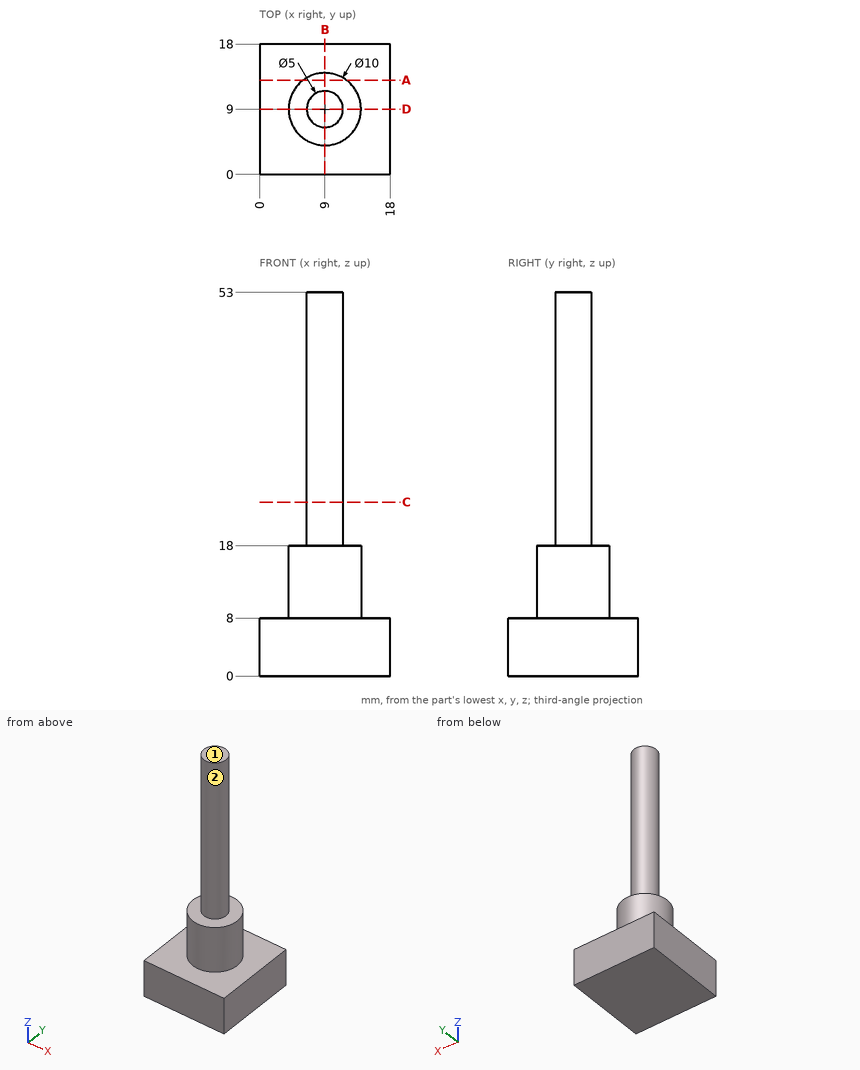
Study the drawing (mm; zero at the part's minimum x, y, z) and answer. A direction names the side the tool comes from. Coordinates: 2 decimals unless noted, no trailing zeros. Loops run counter-clockwise (first coordinate to the right, second up) from the corner with the lowest first, then second, coordinate; pieces in that order, holes last. Notation, with made-up numbers: M -37,-10 L 19,-10 A21 ccw 19,25 Z; hole C -17,16.25 d7. An arc over 180 degrees is marked long. Answer as a JSON object with one key per item and string values. Group by question number.
Item 1: Which of the six approach directions +Z, -Z, +X, -X, +Y, -Y give full straight-line access (tool end or side, diameter ignored) to the marked faces 1 and 2?
Item 2: Section C-C (z = 24) is taken. Write down the section's boundary in (x, y), and give its area (3 significant figures).
Item 3: Section A-A (y = 13) is taken. Write down the section's boundary in (x, z).
Item 4: Each of these flat-tipped pins is pushed along its axis until it touches: P1, Ø4, axis at x = 14, z = 30.5, coming from the +Y side; P2, Ø2, axis at x = 12, z = 15, coming from the -Y side; P3, Ø3, axis at y = 8.5, z = 10, coming from the +X side. Where does it stop, or does it pass through?
Item 5: Section B-B (x = 9) is taken. Write down the section's boundary in (y, z), and give its area (3 significant figures).
Item 6: Consider L1, parallel to Z at x = 10.75, y = 2.5; L2, parallel to Y at x = 9, z = 16; L3, parallel to Z at x = 13.5, y = 8. Determine where each line is inside the solid, lowest interval first.
Solved:
{
 "1": {"face 1": "+Z, +X, -X, +Y, -Y", "face 2": "+Z"},
 "2": {"outline": "C 9,9 d5", "area": "19.6 mm2"},
 "3": {"outline": "M 0,0 L 18,0 L 18,8 L 12,8 L 12,18 L 6,18 L 6,8 L 0,8 Z"},
 "4": {"P1": "passes through", "P2": "stops at y = 4.42", "P3": "stops at x = 14"},
 "5": {"outline": "M 0,0 L 18,0 L 18,8 L 14,8 L 14,18 L 11.5,18 L 11.5,53 L 6.5,53 L 6.5,18 L 4,18 L 4,8 L 0,8 Z", "area": "419 mm2"},
 "6": {"L1": "z = 0 to 8", "L2": "y = 4 to 14", "L3": "z = 0 to 18"}
}
